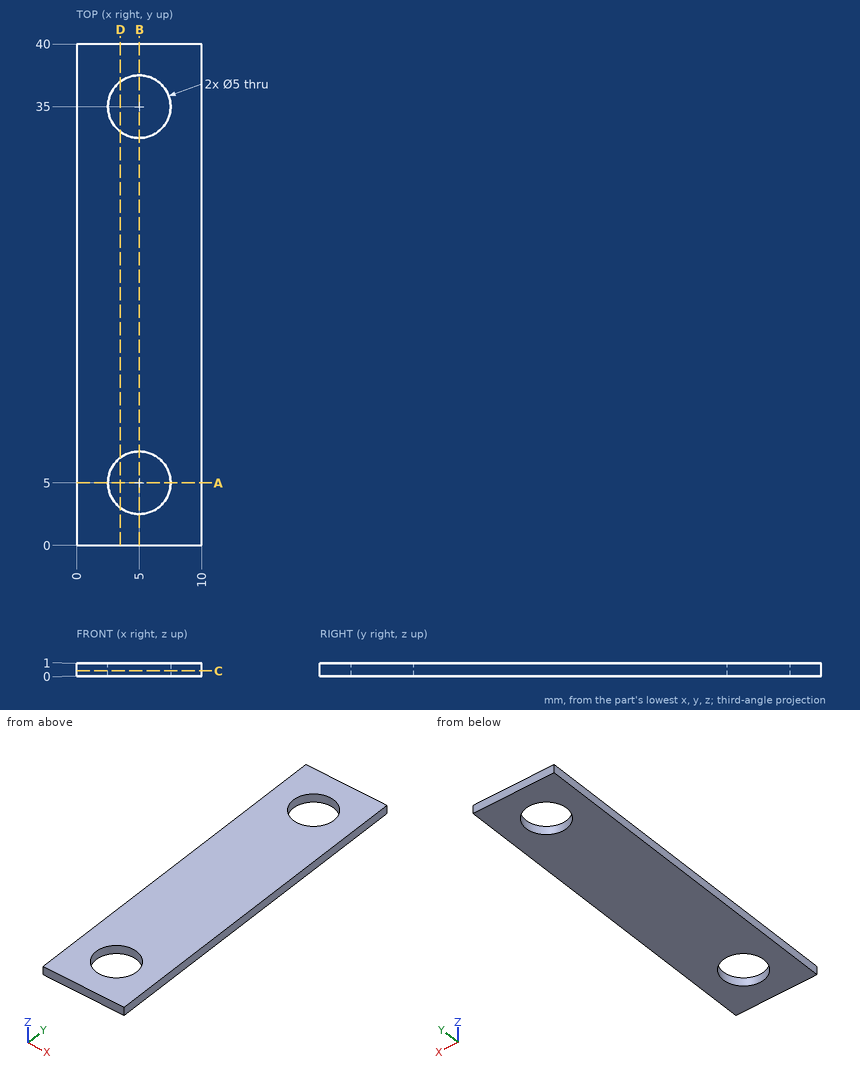
Geometry: see drawing. Coordinates: mm, zero at the bounding-box minimum. Give positions to 0.01 mm unless a question says otherwise; leave off trailing zeros. Loops run counter-clockwise (first coordinate to the right, second up) from the corner with the lowest first, then second, coordinate; pieces in that order, holes last. Notation, with made-up numbers: (50, 77) - (81, 77) arc R20 cw to (81, 98) - close; hole circle Ø10 at (-20.5, -20.5). An arc over 180 degrees is marked (long way). Use CSV: the item, a comma, the result in double quotes. Start each with the question number.
1. Section B-B (x = 5). Output: boundary loops of the cut face in (y, z).
2. Section D-D (x = 3.5). Output: boundary loops of the cut face in (y, z).
3. Ray query, L1, parallel to Y at x = 5, z = 0.55; L2, parallel to X at y = 5, z = 0.4; L3, parallel to Y at x = 3.25, z = 0.2. Return the intervals inside material, ascending.
4. Section C-C (z = 0.4). Output: boundary loops of the cut face in (x, y), then the cut area to 3 significant figures.
5. Section A-A (y = 5). Output: boundary loops of the cut face in (x, z).
Response:
1,outline,"(0, 0) - (2.5, 0) - (2.5, 1) - (0, 1) - close; (7.5, 0) - (32.5, 0) - (32.5, 1) - (7.5, 1) - close; (37.5, 0) - (40, 0) - (40, 1) - (37.5, 1) - close"
2,outline,"(0, 0) - (3, 0) - (3, 1) - (0, 1) - close; (7, 0) - (33, 0) - (33, 1) - (7, 1) - close; (37, 0) - (40, 0) - (40, 1) - (37, 1) - close"
3,L1,"0 to 2.5, 7.5 to 32.5, 37.5 to 40"
3,L2,"0 to 2.5, 7.5 to 10"
3,L3,"0 to 3.21, 6.79 to 33.21, 36.79 to 40"
4,outline,"(0, 0) - (10, 0) - (10, 40) - (0, 40) - close; hole circle Ø5 at (5, 5); hole circle Ø5 at (5, 35)"
4,area,"361 mm²"
5,outline,"(0, 0) - (2.5, 0) - (2.5, 1) - (0, 1) - close; (7.5, 0) - (10, 0) - (10, 1) - (7.5, 1) - close"
